```python
from build123d import *

# Parameters (mm, degrees)
F1_DEPTH = 2.54


with BuildPart() as f1:
    # F0 (on Front) → F1 (new body)
    with BuildSketch(Plane.XZ):
        Polygon((2.113677, 22.124263), (0, 25.4), (-2.113677, 22.124263), (-3.754936, 25.120917), (-5.474462, 21.540216), (-7.919199, 24.133924), (-8.653282, 20.471232), (-11.956969, 22.409616), (-11.956969, 18.734501), (-15.162867, 20.377621), (-15.162867, 16.249249), (-18.59776, 17.299807), (-17.654823, 13.50029), (-21.515161, 13.50029), (-20.103852, 9.475534), (-24.015887, 8.270258), (-21.447383, 5.827554), (-24.991025, 4.539679), (-22.21337, 1.904508), (-22.148459, 1.842926), (-25.4, 0), (-22.148459, -1.842926), (-22.21337, -1.904508), (-24.991025, -4.539679), (-21.447383, -5.827554), (-24.015887, -8.270258), (-20.103852, -9.475534), (-21.515161, -13.50029), (-17.654823, -13.50029), (-18.59776, -17.299807), (-15.162867, -16.249249), (-15.162867, -20.377621), (-11.956969, -18.734501), (-11.956969, -22.409616), (-8.653282, -20.471232), (-7.919199, -24.133924), (-5.474462, -21.540216), (-3.754936, -25.120917), (-2.113677, -22.124263), (0, -25.4), (2.113677, -22.124263), (3.754936, -25.120917), (5.474462, -21.540216), (7.919199, -24.133924), (8.653282, -20.471232), (11.956969, -22.409616), (11.956969, -18.734501), (15.162867, -20.377621), (15.162867, -16.249249), (18.59776, -17.299807), (17.654823, -13.50029), (21.515161, -13.50029), (20.103852, -9.475534), (24.015887, -8.270258), (21.447383, -5.827554), (24.991025, -4.539679), (22.21337, -1.904508), (22.148459, -1.842926), (25.4, 0), (22.148459, 1.842926), (22.21337, 1.904508), (24.991025, 4.539679), (21.447383, 5.827554), (24.015887, 8.270258), (20.103852, 9.475534), (21.515161, 13.50029), (17.654823, 13.50029), (18.59776, 17.299807), (15.162867, 16.249249), (15.162867, 20.377621), (11.956969, 18.734501), (11.956969, 22.409616), (8.653282, 20.471232), (7.919199, 24.133924), (5.474462, 21.540216), (3.754936, 25.120917), align=None)
        Polygon((25.4, 0), (22.21337, 1.904508), (22.148459, 1.842926), align=None)
        Polygon((-22.148459, 1.842926), (-22.21337, 1.904508), (-25.4, 0), align=None)
        Polygon((22.21337, -1.904508), (25.4, 0), (22.148459, -1.842926), align=None)
        Polygon((-22.148459, -1.842926), (-25.4, 0), (-22.21337, -1.904508), align=None)
    extrude(amount=F1_DEPTH)


solid = f1.part
```
Geometry check sheet. Reference: the model listing, model coordinates, mm. A direction names the side the tool comes from. Coordinates: 2 decimals unless noted, no trailing zeros. Order: outer loops, then holes, each group sorted by start corner. A loop starts at its lowest first (then second) coordinate and runs counter-clockwise, first axis right, second up.
Item 1: Section check B-B (z = 3). Enter the section's corners in (x, y), plus the area to 3 significant figures.
Item 2: Tool access check on faces 4 (the flat face through (0, -2.54, 0)), 5 (the flat face through (13.582, -1.252, 19.568)), 6 (the flat face through (-13.582, -1.252, -19.568)), 7 (the flat face through (18.133, -1.252, -15.427)), 8 (the flat face through (-20, -1, -13.5)). Record the directions out of +Z, -Z, +X, -X, +Y, -Y that give a thin tool (end or side, any length) a straight path to the whole face; none if there is none.
Item 3: Mould release check, pull along X, two halves, no side actions. Record for faces 1 (the flat face through (23.78, -1.25, -0.97)), 2 (the flat face through (6.68, -1.25, -22.82)), 3 (the flat face through (-20.8, -1.25, -11.46)): released by +X, released by -X, zero draft, split by the parting line, or undercut.
Item 4: Depth check by flat-ended pin: pin 1 (0.8 mm diameter, centred on y = -0.5, z = -20.5, fed in from -X); pin 2 (1.5 mm diameter, centred on x = 8.5, y = -1.5, fed in from -Z); pin 3 (10 mm diameter, centred on x = 10.5, z = 14.5, fed in from +Y); pin 4 (0.8 mm diameter, centred on x = 18.5, y = -2, fed in from +Z). Enter the tip coordinate at first touch or a pass-through.
Item 5: Section check A-A (x = -19.5). Enter the section's corners in (y, z), plus the area to 3 significant figures.
Item 6: Scan lines: line 1 along X through (y, z) = (-1.5, 22); line 2 along Z through (x, y) = (22.5, -0.2) (3 decimals); line 3 along Z through (x, y) = (20, -1.25). Record each from-to range of solid material in increasing order.
Check sheet entries:
1. outline: (-23.37, -2.54) - (23.37, -2.54) - (23.37, 0) - (-23.37, 0) - close
1. area: 119 mm2
2. face 4: +Z, -Z, +X, -X, -Y
2. face 5: +Z, +Y, -Y
2. face 6: -Z, +Y, -Y
2. face 7: +X, +Y, -Y
2. face 8: -X, +Y, -Y
3. face 1: released by +X
3. face 2: undercut
3. face 3: released by -X
4. pin 1: stops at x = -15.16
4. pin 2: stops at z = -24.13
4. pin 3: stops at y = 0
4. pin 4: stops at z = 17.3
5. outline: (-2.54, -13.5) - (0, -13.5) - (0, 13.5) - (-2.54, 13.5) - close
5. area: 68.6 mm2
6. line 1: x = -11.96 to -11.26, -8.35 to -5.91, -5.25 to 5.25, 5.91 to 8.35, 11.26 to 11.96
6. line 2: z = -8.737 to -6.829, -5.445 to -2.176, -1.733 to 1.733, 2.176 to 5.445, 6.829 to 8.737
6. line 3: z = -13.5 to 13.5
